Part model, mm, in its own coordinate system. A direction names the side the tool comes from. Give positions to 0.01 mm unless a question says otherwise; leave off trailing zeros. Write each loop counter-clockwise with the first axis right and the second up, starting at its lowest first coordinate (ties: lowest second). Pieces come first, ordered by that corner, then holes.
from build123d import *

# Parameters (mm, degrees)
F0_R     = 24
F0_R_2   = 22.5
F1_DEPTH = 2
F3_ANGLE = 35
F4_DEPTH = 2


with BuildPart() as f1:
    # F0 (on Top) → F1 (new body)
    with BuildSketch(Plane.XY):
        Circle(F0_R)
        Circle(F0_R_2, mode=Mode.SUBTRACT)
    extrude(amount=F1_DEPTH)

    # F2 (on Top) → F3 (revolve)
    with BuildSketch(Plane.XY):
        with BuildLine():
            Line((0, 21.5), (0, 24))
            ThreePointArc((0, 24), (-24, 0), (0, -24))
            Line((0, -24), (0, -21.5))
            ThreePointArc((0, -21.5), (-21.5, 0), (0, 21.5))
        make_face()
    revolve(axis=Axis((0, 0, 0), (0, -1, 0)), revolution_arc=F3_ANGLE)

    # F2 (on Top) → F4 (join)
    with BuildSketch(Plane.XY):
        with BuildLine():
            Line((0, 21.5), (0, 24))
            ThreePointArc((0, 24), (-24, 0), (0, -24))
            Line((0, -24), (0, -21.5))
            ThreePointArc((0, -21.5), (-21.5, 0), (0, 21.5))
        make_face()
    extrude(amount=F4_DEPTH)


solid = f1.part
1) 3-axis set-ups, long thin cutter, end or side, ignore diameter. For faces 1 (the flat face through (23, 0, 0)), 2 (the cylindrical face through (-21.495, -0.473, 0.986)): which of +Z, -Z, +X, -X, +Y, -Y reach the whole face in a straight line?
Check result:
face 1: -Z, +X, +Y, -Y
face 2: +Z
2) Flat gauge pins, fed straight in: P1, Ø6, axis at y = -19, z = -6.5, coming from the +X side; P2, Ø8, axis at x = 17, z = -0.5, coming from the -Y side; P3, Ø0.5, axis at y = 22, z = 1.5, coming from the +X side; P4, Ø7, axis at x = 15.5, y = -5, coming from the -Z side. Where does each tip first touch, or does it go through?
Check result:
P1: stops at x = -5.51
P2: stops at y = -20.15
P3: stops at x = 10.15
P4: passes through
3) Mould opens along Y. For faces 3 (the cylindrical face through (22.495, -0.495, 0.986)), 4 (the cylindrical face through (-23.977, 1.055, 0.986)), 5 (the flat face through (-21.4, 3.7, 2)) say: +Y half, -Y half, draft (parallel to the pull), parting line (faces both ways), or undercut.
Check result:
face 3: undercut
face 4: parting line
face 5: draft
4) Saw through at B-B (y = -7). Write the cut outline in (x, z), and give its area (3 significant figures).
Check result:
outline: (-22.96, 0) arc R22.96 ccw to (-18.8, -13.17) - (-16.65, -11.66) arc R20.33 cw to (-20.33, 0) - (-20.33, 2) - (-22.96, 2) - close; (21.38, 0) - (22.96, 0) - (22.96, 2) - (21.38, 2) - close
area: 43.1 mm2
5) Saw through at D-D (y = 19.5). Write the cut outline in (x, z).
Check result:
outline: (-13.99, 0) arc R13.99 ccw to (-11.46, -8.02) - (-7.42, -5.19) arc R9.06 cw to (-9.06, 0) - (-9.06, 2) - (-13.99, 2) - close; (11.22, 0) - (13.99, 0) - (13.99, 2) - (11.22, 2) - close
6) Drill centre lines: L1, parallel to Y at x = -16.5, z = -5.75; L2, parallel to Z at x = 9.5, y = -21; L3, parallel to Y at x = -10.5, z = -5.25. Where is each one in solid material? Low to high.
Check result:
L1: y = -16.45 to -12.53, 12.53 to 16.45
L2: z = 0 to 2
L3: y = -20.93 to -18.01, 18.01 to 20.93
7) Saw through at A-A (x = 10.5). Write the cut outline in (y, z).
Check result:
outline: (-21.58, 0) - (-19.9, 0) - (-19.9, 2) - (-21.58, 2) - close; (19.9, 0) - (21.58, 0) - (21.58, 2) - (19.9, 2) - close
8) Saw through at C-C (x = -14). Write the cut outline in (y, z).
Check result:
outline: (-19.49, 0) arc R19.49 ccw to (-16.85, -9.8) - (-13.04, -9.8) arc R16.32 cw to (-16.32, 0) - (-16.32, 2) - (-19.49, 2) - close; (13.04, -9.8) - (16.85, -9.8) arc R19.49 ccw to (19.49, 0) - (19.49, 2) - (16.32, 2) - (16.32, 0) arc R16.32 cw to start
